Read the model definition and answer for the solid it produces. Units are mm, in the model's axes. Face numbers are marked on the shaded views. Coordinates: 2 decimals unless noted, no trailing zeros. Loops run counter-clockwise (first coordinate to the right, second up) from the corner with the lowest first, then second, coordinate; pieces in that order, holes last. Notation, with made-up numbers: (63, 60.25) -> (116, 60.25) arc R24 cw to (116, 70.25) -> close; hole circle Ø7 at (62, -20.75). An arc over 180 degrees is marked (long way). Answer in a Markdown table with one row per item.
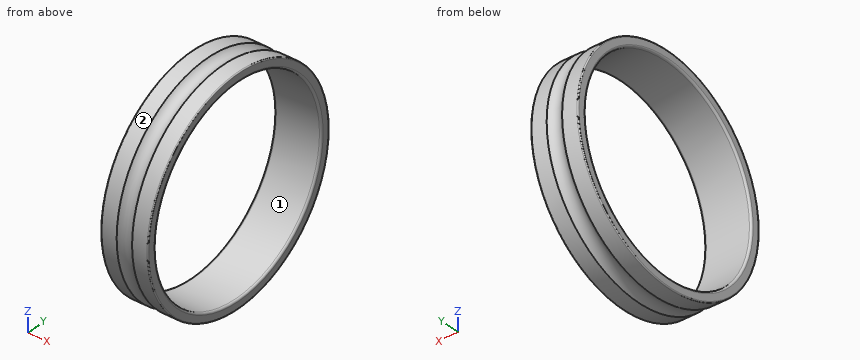
Autodesk Inventor part; units mm, degrees
ref_plane "1_XY" through (1.75, 0, 0) normal (1, 0, 0) x (0, 0, -1)
ref_plane "1_YZ" through (1.75, 0, 0) normal (0, 0, -1) x (0, 1, 0)
ref_plane "1_ZX" through (1.75, 0, 0) normal (0, 1, 0) x (1, 0, 0)
sketch "Sketch_1" plane through (0, 0, 0) normal (0, 0, 1) x (1, 0, 0)
  line L0 (3.5, 0) -> (0, 0)
  line L1 (0, 8.125) -> (0, 7.65)
  arc A0 (0, 7.65) -> (0.15, 7.5) centre (0.15, 7.65) ccw
  line L2 (0.15, 7.5) -> (3.35, 7.5)
  arc A1 (3.35, 7.5) -> (3.5, 7.65) centre (3.35, 7.65) ccw
  line L3 (3.5, 7.65) -> (3.5, 8.125)
  arc A2 (3.5, 8.125) -> (3.425, 8.2) centre (3.425, 8.125) ccw
  line L4 (3.425, 8.2) -> (2.3223, 8.2)
  arc A3 (1.1777, 8.2) -> (2.3223, 8.2) centre (1.75, 8.75) ccw
  line L5 (1.1777, 8.2) -> (0.075, 8.2)
  arc A4 (0.075, 8.2) -> (0, 8.125) centre (0.075, 8.125) ccw
revolve "Revolution1" add sketch "Sketch_1" angle 360 about axis through (3.5, 0, 0) along (1, 0, 0)
ref_plane "1_XY" through (1.75, 0, 0) normal (1, 0, 0) x (0, 0, -1)
ref_plane "1_YZ" through (1.75, 0, 0) normal (0, 0, -1) x (0, 1, 0)
ref_plane "1_ZX" through (1.75, 0, 0) normal (0, 1, 0) x (1, 0, 0)
ref_plane "1_Dummy_XY" through (0, 0, 0) normal (-1, 0, 0) x (0, 0, -1)
ref_plane "1_Dummy_YZ" through (0, 0, 0) normal (0, 0, -1) x (0, -1, 0)
ref_plane "1_Dummy_ZX" through (0, 0, 0) normal (0, -1, 0) x (-1, 0, 0)
properties part number "A-2015_ir"
1. A cutting plane is placed at A-A on z = 0. Give the vertices of the cut face in (x, y) (3 decimals).
A:
| item | result |
|---|---|
| outline | (0, -8.125) arc R0.075 ccw to (0.075, -8.2) -> (1.178, -8.2) arc R0.794 cw to (2.322, -8.2) -> (3.425, -8.2) arc R0.075 ccw to (3.5, -8.125) -> (3.5, -7.65) arc R0.15 ccw to (3.35, -7.5) -> (0.15, -7.5) arc R0.15 ccw to (0, -7.65) -> close; (0, 7.65) arc R0.15 ccw to (0.15, 7.5) -> (3.35, 7.5) arc R0.15 ccw to (3.5, 7.65) -> (3.5, 8.125) arc R0.075 ccw to (3.425, 8.2) -> (2.322, 8.2) arc R0.794 cw to (1.178, 8.2) -> (0.075, 8.2) arc R0.075 ccw to (0, 8.125) -> close |
2. Given pin 1 Ø1 at (x, y) = (3, -3.5) entering from +Z; pin 2 Ø6 at (y, z) = (-6, -2.5) entering from -X; pin 3 Ø1.5 at (x, y) = (1, -6) entering from +Z; pin 4 Ø1 at (x, y) = (2, -5) entering from +Z, each flat-ended and moving along its own axis, determine where each tip first touches the part or whether it passes through.
A:
| item | result |
|---|---|
| pin 1 | stops at z = 7.63 |
| pin 2 | stops at x = 0 |
| pin 3 | stops at z = 6.3 |
| pin 4 | stops at z = 6.78 |
3. Find the intervals of material crossed by probe 1 along Z at (x, y) = (2.4, 0); probe 2 along Y at (x, z) = (2.3, 3); probe 3 along Z at (x, y) = (2.35, -3.5), in increasing order.
A:
| item | result |
|---|---|
| probe 1 | z = -8.2 to -7.5, 7.5 to 8.2 |
| probe 2 | y = -7.61 to -6.87, 6.87 to 7.61 |
| probe 3 | z = -7.42 to -6.63, 6.63 to 7.42 |
4. A cutting plane is placed at C-C on x = 3. Give the vertices of the cut face in (y, z), and give its area (3 significant figures).
A:
| item | result |
|---|---|
| outline | circle Ø16.4 at (0, 0); hole circle Ø15 at (0, 0) |
| area | 34.5 mm2 |
5. The mould has two halves that part along Y. Classify the marked faces 1 and 2: pulls with the +Y half, pulls with the -Y half, needs draft (parallel to the pull), parting line crosses it, or undercut.
A:
| item | result |
|---|---|
| face 1 | undercut |
| face 2 | parting line crosses it |
